Source: CAD feature listing. Evaluate the final solid. Frame: model axes, mm. Face numbers are marked on the shaded views. Round coordinates to 2 decimals unless told otherwise and drop trailing zeros. Write each loop counter-clockwise with the first axis right and the second up, starting at its lowest first coordinate (ties: lowest second). Pieces come first, ordered by that corner, then holes.
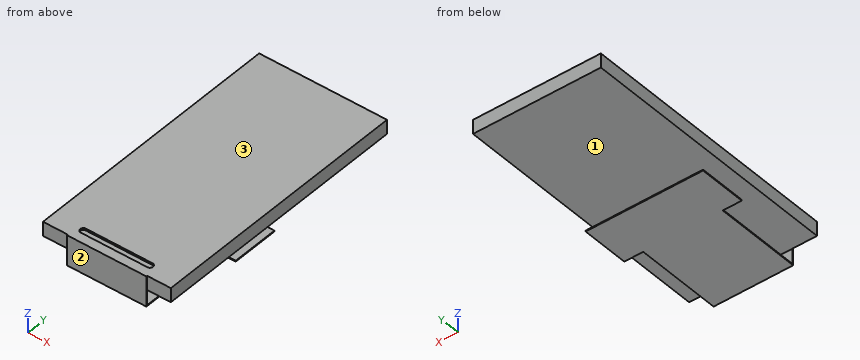
from build123d import *

# Parameters (mm, degrees)
SKETCH_W        = 10.8
SKETCH_H        = 21.7
PAD_DEPTH       = 0.5
SKETCH001_W     = 12.8
SKETCH001_H     = 24.6
PAD001_DEPTH    = 0.6
SKETCH002_W     = 13.5
SKETCH002_H     = 27.95
PAD002_DEPTH    = 1.5
SKETCH003_W     = 8.4
SKETCH003_H     = 1.5
PAD003_DEPTH    = 0.1
PAD003_FACE10_W = 0.1
PAD003_FACE10_H = 8.4
PAD004_DEPTH    = 1.7
SKETCH005_W     = 8.4
SKETCH005_H     = 0.1
PAD005_DEPTH    = 14
SKETCH006_W     = 12.4
SKETCH006_H     = 5
PAD006_DEPTH    = 0.1
POCKET_DEPTH    = 0.2


with BuildPart() as part:
    # Sketch → Pad (new body)
    with BuildSketch(Plane.XY):
        Rectangle(SKETCH_W, SKETCH_H)
    extrude(amount=PAD_DEPTH)

    # Sketch001 (on Face6 of Pad) → Pad001 (join)
    with BuildSketch(Plane.XY.offset(0.5)):
        Rectangle(SKETCH001_W, SKETCH001_H)
    extrude(amount=-PAD001_DEPTH)

    # Sketch002 (on Face4 of Pad001) → Pad002 (join)
    with BuildSketch(Plane.XY.offset(0.5)):
        with Locations((-0.05, -0.775)):
            Rectangle(SKETCH002_W, SKETCH002_H)
    extrude(amount=-PAD002_DEPTH)

    # Sketch003 (on Face6 of Pad002) → Pad003 (join)
    with BuildSketch(Plane.XZ.offset(14.75)):
        with Locations((0, -0.25)):
            Rectangle(SKETCH003_W, SKETCH003_H)
    extrude(amount=PAD003_DEPTH)

    # Pad003 Face10 → Pad004 (add)
    with BuildSketch(Plane(origin=(0, -14.8, -1), x_dir=(0, -1, 0), z_dir=(0, 0, -1))):
        Rectangle(PAD003_FACE10_W, PAD003_FACE10_H)
    extrude(amount=PAD004_DEPTH)

    # Sketch005 (on Face10 of Pad004) → Pad005 (join)
    with BuildSketch(Plane(origin=(0, -14.75, 0), x_dir=(-1, 0, 0), z_dir=(0, 1, 0))):
        with Locations((0, -2.65)):
            Rectangle(SKETCH005_W, SKETCH005_H)
    extrude(amount=PAD005_DEPTH)

    # Sketch006 (on Face23 of Pad005) → Pad006 (join)
    with BuildSketch(Plane(origin=(0, 0, -2.7), x_dir=(1, 0, 0), z_dir=(0, 0, -1))):
        with Locations((0, 3.25)):
            Rectangle(SKETCH006_W, SKETCH006_H)
    extrude(amount=-PAD006_DEPTH)

    # Sketch007 (on Face4 of Pad006) → Pocket (cut)
    with BuildSketch(Plane.XY.offset(0.5)):
        with BuildLine():
            ThreePointArc((-3.515, -13.22), (-3.845, -13.55), (-3.515, -13.88))
            Line((-3.515, -13.88), (3.515, -13.88))
            ThreePointArc((3.515, -13.88), (3.845, -13.55), (3.515, -13.22))
            Line((3.515, -13.22), (-3.515, -13.22))
        make_face()
    extrude(amount=-POCKET_DEPTH, mode=Mode.SUBTRACT)


solid = part.part
1) Material intervals for line 1 (Y direction, x = 5.5, z = 0.15); line 2 (Z direction, x = 1.25, y = 9), sorted ascending.
Taken from the geometry:
line 1: y = -14.75 to 13.2
line 2: z = -1 to 0.5
2) Contact query for flat-ended pins moving along their axis: P1, Ø0.5, axis at x = 0, z = -1.5, coming from the +Y side; P2, Ø1.5, axis at x = -5, z = -2.5, coming from the -Y side; P3, Ø1.6, axis at x = 5.5, z = 0, coming from the -Y side. Output: stop coordinate, or through.
Taken from the geometry:
P1: stops at y = -14.75
P2: stops at y = -5.75
P3: stops at y = -14.75
3) Section query C-C on y = -13.55. Return the cut outline in (x, z) (3 decimals), then the cut area to 3 significant figures.
Taken from the geometry:
outline: (-6.8, -1) - (6.7, -1) - (6.7, 0.5) - (3.845, 0.5) - (3.845, 0.3) - (-3.845, 0.3) - (-3.845, 0.5) - (-6.8, 0.5) - close; (-4.2, -2.7) - (4.2, -2.7) - (4.2, -2.6) - (-4.2, -2.6) - close
area: 19.6 mm2
4) Section query A-A on y = -10. Return the cut outline in (x, z), then the cut area to 3 significant figures.
Taken from the geometry:
outline: (-6.8, -1) - (6.7, -1) - (6.7, 0.5) - (-6.8, 0.5) - close; (-4.2, -2.7) - (4.2, -2.7) - (4.2, -2.6) - (-4.2, -2.6) - close
area: 21.1 mm2
5) Pull-direction query (Z, two-part tool) for the marked faces 1, 2 and 3; classes: released by +Z, released by -Z, zero draft, split by the parting line, or undercut.
Taken from the geometry:
face 1: undercut
face 2: zero draft
face 3: released by +Z
6) Section query B-B on x = 4.75. Return the cut outline in (y, z).
Taken from the geometry:
outline: (-14.75, -1) - (13.2, -1) - (13.2, 0.5) - (-14.75, 0.5) - close; (-5.75, -2.7) - (-0.75, -2.7) - (-0.75, -2.6) - (-5.75, -2.6) - close
7) Section query D-D on z = -1.5. Return the cut outline in (x, y).
Taken from the geometry:
outline: (-4.2, -14.85) - (4.2, -14.85) - (4.2, -14.75) - (-4.2, -14.75) - close
